```python
from build123d import *

# Parameters (mm, degrees)
F0_W     = 26
F0_H     = 30
F0_W_2   = 22
F0_H_2   = 26
F1_DEPTH = 17
F2_DEPTH = 2
F3_W     = 19
F3_H     = 28
F3_W_2   = 15
F3_H_2   = 24
F4_DEPTH = 10


with BuildPart() as f1:
    # F0 (on Top) → F1 (new body)
    with BuildSketch(Plane.XY):
        Rectangle(F0_W, F0_H)
        Rectangle(F0_W_2, F0_H_2, mode=Mode.SUBTRACT)
    extrude(amount=-F1_DEPTH)

    # F0 (on Top) → F2 (join)
    with BuildSketch(Plane.XY):
        Rectangle(F0_W_2, F0_H_2)
    extrude(amount=-F2_DEPTH)

    # F3 (on Top) → F4 (join)
    with BuildSketch(Plane.XY):
        with Locations((-2.5, 0)):
            Rectangle(F3_W, F3_H)
        with Locations((-2.5, 0)):
            Rectangle(F3_W_2, F3_H_2, mode=Mode.SUBTRACT)
    extrude(amount=F4_DEPTH)


solid = f1.part
```
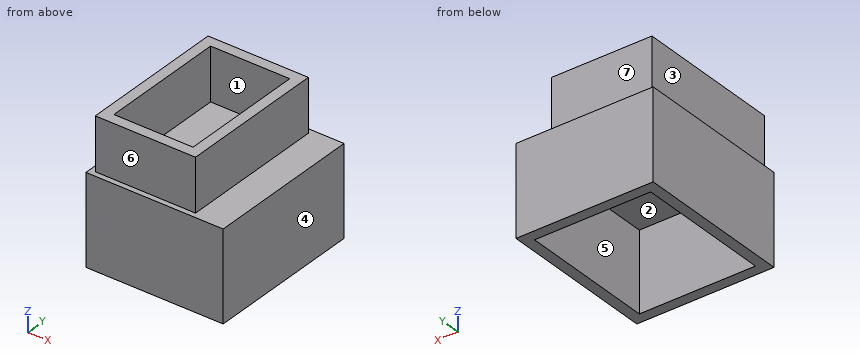
Geometry check sheet. Reference: the model listing, model coordinates, mm. Face numbers are marked on the shaded views. A direction names the side the tool comes from. Coordinates: 2 decimals unless noted, no trailing zeros. Loops run counter-clockwise (first coordinate to the right, second up) from the corner with the lowest first, then second, coordinate; pieces in that order, holes last. Notation, with made-up numbers: (-16.75, -22) - (26.25, -22) arc R18 cw to (26.25, -13) - close; hole circle Ø7 at (-21.5, 28). An arc over 180 degrees is marked (long way). One line per item, written item: value. Start each with the question number.
(1) Cross-section at B-B on x = 10.5. Enter the section's corners in (y, z).
(2) Cross-section at A-A on z = -14.75. Enter the section's corners in (x, y), plus the area to 3 significant figures.
(3) Cross-section at C-C on y = -12.5. Enter the section's corners in (x, z), plus the area to 3 significant figures.
(4) Tool access check on the marked faces 1, 2 and 3. Record the directions out of +Z, -Z, +X, -X, +Y, -Y that give a thin tool (end or side, any length) a straight path to the whole face; none if there is none.
(5) Depth check by flat-ended pin: P1, Ø5, axis at y = 4, z = 5, coming from the -X side; P2, Ø10, axis at x = -9, y = 4.5, coming from the -Z side; P3, Ø3, axis at x = -0.5, y = -1, coming from the -Z side; P4, Ø5, axis at x = 0.5, z = 6.5, coming from the +Y side. Enter the tip coordinate at first touch or a pass-through.
(6) Material ranges on line 1 (Y direction, x = -6.5, z = -14); line 2 (X direction, y = -5, z = 5.25); line 3 (X direction, y = -2.75, z = -2.75), recorded low to high. Write a range as [from, to].
(7) Cross-section at D-D on z = 6.75. Enter the section's corners in (x, y).
(8) Mould release check, pull along Y, two halves, no side actions. Record for the marked faces 4, 5, 6 and 7: released by +Y, released by -Y, zero draft, split by the parting line, or undercut.
Results below:
1. outline: (-15, -17) - (-13, -17) - (-13, -2) - (13, -2) - (13, -17) - (15, -17) - (15, 0) - (-15, 0) - close
2. outline: (-13, -15) - (13, -15) - (13, 15) - (-13, 15) - close; hole (-11, -13) - (11, -13) - (11, 13) - (-11, 13) - close
2. area: 208 mm2
3. outline: (-13, -17) - (-11, -17) - (-11, -2) - (11, -2) - (11, -17) - (13, -17) - (13, 0) - (7, 0) - (7, 10) - (-12, 10) - (-12, 0) - (-13, 0) - close
3. area: 302 mm2
4. face 1: +Z
4. face 2: -Z
4. face 3: +Z, -X, +Y, -Y
5. P1: stops at x = -12
5. P2: stops at z = -17
5. P3: stops at z = -2
5. P4: stops at y = 14
6. line 1: y = [-15, -13], [13, 15]
6. line 2: x = [-12, -10], [5, 7]
6. line 3: x = [-13, -11], [11, 13]
7. outline: (-12, -14) - (7, -14) - (7, 14) - (-12, 14) - close; hole (-10, -12) - (5, -12) - (5, 12) - (-10, 12) - close
8. face 4: zero draft
8. face 5: undercut
8. face 6: released by -Y
8. face 7: released by +Y
